```python
from build123d import *

# Parameters (mm, degrees)
SKETCH_1_W      = 200
SKETCH_1_H      = 150
EXTRUDE_1_DEPTH = 5
SKETCH_2_W      = 20
SKETCH_2_H      = 20
SKETCH_2_R      = 6.054352045
EXTRUDE_2_DEPTH = 5
FILLET_1_R      = 10


with BuildPart() as part:
    # 草图1 → 凸台-拉伸1 (new body)
    with BuildSketch(Plane.XY):
        Rectangle(SKETCH_1_W, SKETCH_1_H)
    extrude(amount=EXTRUDE_1_DEPTH)

    # 草图2 → 凸台-拉伸2 (add)
    # profile 1 of 2: a face of its own
    with BuildSketch(Plane.XY):
        with Locations((-110, 0.621152281)):
            Rectangle(SKETCH_2_W, SKETCH_2_H)
        with Locations((-110.38820767, 0)):
            Circle(SKETCH_2_R, mode=Mode.SUBTRACT)
    # profile 2 of 2: a face of its own
    with BuildSketch(Plane.XY):
        with Locations((110, 0.621152281)):
            Rectangle(SKETCH_2_W, SKETCH_2_H)
        with Locations(Location((110.38820767, 0, 0), (0, 0, 180))):
            Circle(SKETCH_2_R, mode=Mode.SUBTRACT)
    extrude(amount=EXTRUDE_2_DEPTH)

    # 圆角1
    fillet_1_edges = [part.edges().sort_by_distance(p)[0] for p in [
        (120, -9.378847719, 2.5),
        (120, 10.621152281, 2.5),
        (-120, -9.378847719, 2.5),
        (-120, 10.621152281, 2.5),
    ]]
    fillet(fillet_1_edges, radius=FILLET_1_R - 0.0001)  # a hair under: the kernel refuses the full size


solid = part.part
```
For this review, take the finished solid that the model builds, in its own axes (mm). A direction names the side the tool comes from. Coordinates: 2 decimals unless noted, no trailing zeros. Order: outer loops, then holes, each group sorted by start corner. A loop starts at its lowest first (then second) coordinate and runs counter-clockwise, first axis right, second up. Notation, with made-up numbers: (57, -24.75) -> (84, -24.75) arc R19 ccw to (84, -17.75) -> close; hole circle Ø3 at (79, 48). An arc over 180 degrees is marked (long way). Use CSV: the item, a comma, the result in double quotes. Start each with the question number.
Item 1: Wall thickness on probe 1 along X at (y, z) = (-22.5, 3.3); probe 2 along Y at (x, z) = (107.5, 2.1): over which ranges is each line inside the solid? List them lowest first.
Item 2: For faces 4 (the face through (-105, 10.621, 2)), 5 (the face through (100, 42, 2)), 6 (the face through (105, -9.379, 2)), 7 (the face through (-1, 75, 2)), 8 (the face through (-105, -9.379, 2)), list the 3-axis set-ups (+Z, -Z, +X, -X, +Y, -Y) from which the entire face can be reached by the end or side of a thin tool; tool diameter is ignored.
Item 3: Draft analysis for pull direction X (two halves, no side actions). For faces 1 (the face through (-100, 42, 2)), 2 (the face through (-2, 1, 5)), 3 (the face through (-104.796, -2.319, 2.465)), state which applies: pulls with the +X half, pulls with the -X half, needs draft (parallel to the pull), parting line crosses it, or undercut.
Item 4: We need section A-A, the plane y = -46. Give the boundary of the cut face in (x, z), then the cut area to 3 significant figures.
Item 5: Insertion check: pin 1 (1.5 mm diameter, centred on y = -40, z = 2, fed in from -X); pin 2 (1 mm diameter, centred on y = 47, z = 2.5, fed in from +X); pin 3 (1.5 mm diameter, centred on x = 107, z = 2.5, fed in from +Y). Each pin has a flat end and moves straight along its axis. Give the tip position at first contact, or say it passes through.
Derived:
1,probe 1,"x = -100 to 100"
1,probe 2,"y = -9.38 to -5.32, 5.32 to 10.62"
2,face 4,"+Z, -Z, -X, +Y"
2,face 5,"+Z, -Z, +X, +Y"
2,face 6,"+Z, -Z, +X, -Y"
2,face 7,"+Z, -Z, +X, -X, +Y"
2,face 8,"+Z, -Z, -X, -Y"
3,face 1,"pulls with the -X half"
3,face 2,"needs draft"
3,face 3,"undercut"
4,outline,"(-100, 0) -> (100, 0) -> (100, 5) -> (-100, 5) -> close"
4,area,"1,000 mm^2"
5,pin 1,"stops at x = -100"
5,pin 2,"stops at x = 100"
5,pin 3,"stops at y = 10.62"
